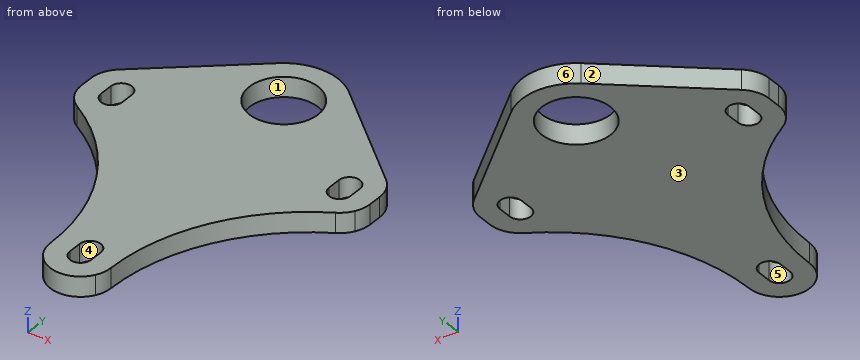
Autodesk Inventor part; units mm, degrees
ref_plane "YZ Plane" through (0, 0, 0) normal (1, 0, 0) x (0, 1, 0)
ref_plane "XZ Plane" through (0, 0, 0) normal (0, 1, 0) x (-1, 0, 0)
ref_plane "XY Plane" through (0, 0, 0) normal (0, 0, 1) x (1, 0, 0)
sketch "スケッチ1" plane through (0, 0, 0) normal (0, 0, 1) x (1, 0, 0)
  circle A0 centre (0, 0) radius 5.2
  line L0 (25, -50) -> (-25, -50)
  line L1 (-25, -50) -> (-25, 50)
  line L2 (-25, 50) -> (25, 50)
  line L3 (25, 50) -> (25, -50)
  line L4 (25, -50) -> (-25, 50) construction
  line L5 (-25, -50) -> (25, 50) construction
  dimension "d0" = 10.4
  dimension "d1" = 50
  dimension "d2" = 100
extrude "押し出し1" add sketch "スケッチ1" along normal blind 3
sketch "スケッチ2" plane through (0, 0, 3) normal (0, 0, 1) x (1, 0, 0)
  circle A0 centre (17.3198, -9.9987) radius 1.25 construction
  circle A1 centre (-17.3213, -10.0013) radius 1.25 construction
  circle A2 centre (0.0015, -40) radius 1.25 construction
  line L0 (-17.3213, -10.0013) -> (-17.3213, -12.0013) construction
  line L1 (-18.9213, -10.0013) -> (-18.9213, -12.0013)
  line L2 (-15.7213, -12.0013) -> (-15.7213, -10.0013)
  arc A3 (-15.7213, -10.0013) -> (-18.9213, -10.0013) centre (-17.3213, -10.0013) ccw
  arc A4 (-18.9213, -12.0013) -> (-15.7213, -12.0013) centre (-17.3213, -12.0013) ccw
  line L3 (0.0015, -40) -> (0.0015, -42) construction
  line L4 (-1.5985, -40) -> (-1.5985, -42)
  line L5 (1.6015, -42) -> (1.6015, -40)
  arc A5 (1.6015, -40) -> (-1.5985, -40) centre (0.0015, -40) ccw
  arc A6 (-1.5985, -42) -> (1.6015, -42) centre (0.0015, -42) ccw
  line L6 (17.3198, -9.9987) -> (17.3198, -11.9987) construction
  line L7 (15.7198, -9.9987) -> (15.7198, -11.9987)
  line L8 (18.9198, -11.9987) -> (18.9198, -9.9987)
  arc A7 (18.9198, -9.9987) -> (15.7198, -9.9987) centre (17.3198, -9.9987) ccw
  arc A8 (15.7198, -11.9987) -> (18.9198, -11.9987) centre (17.3198, -11.9987) ccw
  circle A9 centre (0, 0) radius 5.2
  arc A10 (5.3111, 6.2476) -> (-5.3114, 6.2473) centre (0, 0) ccw
  line L9 (-12.7213, -12.0013) -> (-12.7213, -10.0013)
  arc A11 (-20.3008, -6.4967) -> (-21.9213, -10.0013) centre (-17.3213, -10.0013) ccw
  line L10 (-21.9213, -10.0013) -> (-21.9213, -12.0013)
  arc A12 (-21.9213, -12.0013) -> (-21.3048, -14.3016) centre (-17.3213, -12.0013) ccw
  line L11 (21.9198, -11.9987) -> (21.9198, -9.9987)
  arc A13 (21.9198, -9.9987) -> (20.2992, -6.494) centre (17.3198, -9.9987) ccw
  line L12 (12.7198, -9.9987) -> (12.7198, -11.9987)
  arc A14 (21.3037, -14.2984) -> (21.9198, -11.9987) centre (17.3198, -11.9987) ccw
  line L13 (4.6015, -40) -> (4.6015, -42)
  arc A15 (-3.9821, -44.3003) -> (3.9854, -44.2997) centre (0.0015, -42) ccw
  line L14 (-4.5985, -42) -> (-4.5985, -40)
  arc A16 (4.6015, -40) -> (-4.5985, -40) centre (0.0015, -40) ccw
  line L15 (-20.3008, -6.4967) -> (-5.3114, 6.2473)
  line L16 (5.3111, 6.2476) -> (20.2992, -6.494)
  line L17 (21.3037, -14.2984) -> (3.9854, -44.2997)
  line L18 (-3.9821, -44.3003) -> (-21.3048, -14.3016)
  point P0 (-17.3213, -11.0013)
  point P1 (0.0015, -41)
  point P2 (17.3198, -10.9987)
  dimension "d5" = 1.6
  dimension "d6" = 2
  dimension "d7" = 3
  dimension "d8" = 3
  dimension "d9" = 3
  dimension "d10" = 3
extrude "押し出し2" cut sketch "スケッチ2" against normal blind 3 keep common part
sketch "スケッチ3" plane through (0, 0, 3) normal (0, 0, 1) x (1, 0, 0)
  arc A0 (15.7198, -11.9987) -> (18.9198, -11.9987) centre (17.3198, -11.9987) ccw
  line L0 (15.7198, -9.9987) -> (15.7198, -11.9987)
  arc A1 (18.9198, -9.9987) -> (15.7198, -9.9987) centre (17.3198, -9.9987) ccw
  line L1 (18.9198, -11.9987) -> (18.9198, -9.9987)
  arc A2 (-1.5985, -42) -> (1.6015, -42) centre (0.0015, -42) ccw
  line L2 (-1.5985, -40) -> (-1.5985, -42)
  arc A3 (1.6015, -40) -> (-1.5985, -40) centre (0.0015, -40) ccw
  line L3 (1.6015, -42) -> (1.6015, -40)
  arc A4 (-18.9213, -12.0013) -> (-15.7213, -12.0013) centre (-17.3213, -12.0013) ccw
  line L4 (-18.9213, -10.0013) -> (-18.9213, -12.0013)
  arc A5 (-15.7213, -10.0013) -> (-18.9213, -10.0013) centre (-17.3213, -10.0013) ccw
  line L5 (-15.7213, -12.0013) -> (-15.7213, -10.0013)
  line L6 (-21.9213, -12.0013) -> (-21.9213, -10.0013)
  arc A6 (-21.9213, -12.0013) -> (-21.3048, -14.3016) centre (-17.3213, -12.0013) ccw
  line L7 (-3.9821, -44.3003) -> (-21.3048, -14.3016)
  arc A7 (-3.9821, -44.3003) -> (3.9854, -44.2997) centre (0.0015, -42) ccw
  line L8 (21.3037, -14.2984) -> (3.9854, -44.2997)
  arc A8 (21.3037, -14.2984) -> (21.9198, -11.9987) centre (17.3198, -11.9987) ccw
  line L9 (21.9198, -9.9987) -> (21.9198, -11.9987)
  arc A9 (21.9198, -9.9987) -> (20.2992, -6.494) centre (17.3198, -9.9987) ccw
  line L10 (5.3111, 6.2476) -> (20.2992, -6.494)
  arc A10 (5.3111, 6.2476) -> (-5.3114, 6.2473) centre (0, 0) ccw
  line L11 (-20.3008, -6.4967) -> (-5.3114, 6.2473)
  arc A11 (-20.3008, -6.4967) -> (-21.9213, -10.0013) centre (-17.3213, -10.0013) ccw
  circle A12 centre (0, 0) radius 5.2
  arc A13 (19.6173, -15.9838) -> (4.6015, -41.9965) centre (34.6015, -41.9737) ccw
  arc A14 (19.6173, -15.9838) -> (21.3037, -14.2984) centre (17.3198, -11.9987) ccw
  arc A15 (-21.3048, -14.3016) -> (-19.6182, -15.9868) centre (-17.3213, -12.0013) ccw
  arc A16 (-4.5985, -41.9972) -> (-19.6182, -15.9868) centre (-34.5985, -41.9789) ccw
  arc A17 (-4.5985, -41.9972) -> (-3.9821, -44.3003) centre (0.0015, -42) ccw
  arc A18 (3.9854, -44.2997) -> (4.6015, -41.9965) centre (0.0015, -42) ccw
  arc A19 (-21.9213, -12.0013) -> (-21.3048, -14.3016) centre (-17.3213, -12.0013) ccw
  dimension "d14" = 30
extrude "押し出し3" cut sketch "スケッチ3" against normal through all contours L6 A11 L11 A10 L10 A9 L9 A8 A14 A13 A18 A7 A17 A16 A15 A6 keep common part
properties part number "POTplate" material "アルミニウム 2014-T4"
Here's how the part is built. I have some questions about the finished solid (model axes, mm). Face numbers are marked on the shaded views. A direction names the side the tool comes from. Give positions to 0.01 mm unless a question says otherwise; leave off trailing zeros. Write each loop counter-clockwise with the first axis right and the second up, starting at its lowest first coordinate (ties: lowest second). Pieces come first, ordered by that corner, then holes. Notation, with made-up numbers: (49, 44) -> (70, 44) arc R4 cw to (70, 50) -> close; hole circle Ø3 at (3, 84). An arc over 180 degrees is marked (long way). Use one line per item in the form item = value.
1) I'm going to push flat-ended pins straight in: pin 1 (1.6 mm diameter, centred on y = -41, z = 2, fed in from -X); pin 2 (1 mm diameter, centred on y = -41.5, z = 1, fed in from +X). Where does each tip first touch, or does it pass through?
Verdict:
pin_1 = -4.65
pin_2 = 4.62
2) If I drill on L1, parallel to Y at x = 0, z = 1.55; L2, parallel to X at y = -1, z = 0.5; L3, parallel to X at y = -39, z = 2.2, over which ranges is the centre line in solid material (lowest first)? Write a range as [from, to].
Verdict:
L1 = [-46.6, -43.6], [-38.4, -5.2], [5.2, 8.2]
L2 = [-13.84, -5.1], [5.1, 13.84]
L3 = [-4.75, -1.25], [1.25, 4.75]
3) Suppose I cut it at A-A (x = 0). Please give me the cut outline in (y, z), and give its area (3 significant figures).
Verdict:
outline = (-46.6, 0) -> (-43.6, 0) -> (-43.6, 3) -> (-46.6, 3) -> close; (-38.4, 0) -> (-5.2, 0) -> (-5.2, 3) -> (-38.4, 3) -> close; (5.2, 0) -> (8.2, 0) -> (8.2, 3) -> (5.2, 3) -> close
area = 118 mm2
4) Suppose I cut it at D-D (x = -11.5). Please give me the cut outline in (y, z).
Verdict:
outline = (-22.84, 0) -> (0.99, 0) -> (0.99, 3) -> (-22.84, 3) -> close
5) Suppose I cut it at B-B (z = 0.7). Give the number of separate pieces and of enclosed holes in the cut face, and give its area (3 significant figures).
Verdict:
separate_pieces = 1
enclosed_holes = 4
area = 1,120 mm2
6) Suppose I cut it at C-C (y = 0). Please give me the cut outline in (x, z), and give its area (3 significant figures).
Verdict:
outline = (-12.66, 0) -> (-5.2, 0) -> (-5.2, 3) -> (-12.66, 3) -> close; (5.2, 0) -> (12.66, 0) -> (12.66, 3) -> (5.2, 3) -> close
area = 44.8 mm2
7) We'd pull the mould along Y, two halves only. Please class the marked faces 1, 2, 3 and 4: +Y half, -Y half, draft (parallel to the pull), parting line (faces both ways), or undercut.
Verdict:
face_1 = undercut
face_2 = +Y half
face_3 = draft
face_4 = undercut
8) On a 3-axis mill with a long thin cutter (end or side, diameter ignored), from which of +Z, -Z, +X, -X, +Y, -Y can I reach the whole of each face in a straight line? I mean the marked faces 5 and 6. Say none if no direction works.
Verdict:
face_5 = +Z, -Z
face_6 = +Z, -Z, +Y
